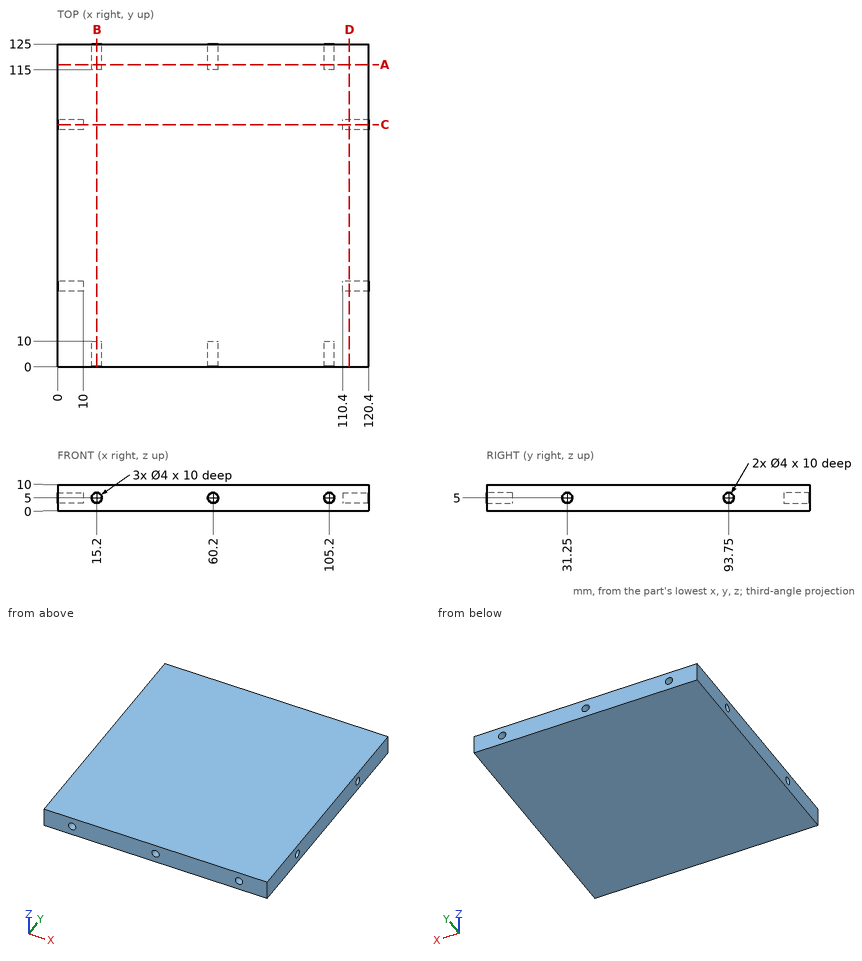
Could you check a few things on this drawing? It's one solid part, dimensions in mm from its lowest x, y, z. Give positions to 0.01 mm unless a question says otherwise; leave off trailing zeros. Write each loop counter-clockwise with the first axis right and the second up, starting at its lowest first coordinate (ties: lowest second). Pieces come first, ordered by that corner, then holes. Notation, with made-up numbers: (71, 0.25) -> (80, 0.25) arc R13 cw to (80, 22.25) -> close; hole circle Ø5 at (53.25, 78.5). An arc over 180 degrees is marked (long way). Answer as a JSON object with one key per item and string values.
Q1. Suppose I cut it at B-B on x = 15.2. Write out the boundary of the cut face in (y, z).
Taken from the geometry:
{"outline": "(0, 0) -> (125, 0) -> (125, 3) -> (115, 3) -> (115, 7) -> (125, 7) -> (125, 10) -> (0, 10) -> (0, 7) -> (10, 7) -> (10, 3) -> (0, 3) -> close"}
Q2. Will these pins go through, and if not, where does the flat tip stop? pin 1 Ø1.2 at (x, z) = (14.5, 4.5) entering from -Y; pin 2 Ø2 at (y, z) = (93, 4.5) entering from -X; pin 3 Ø1.2 at (x, z) = (106, 5.5) entering from +Y.
Taken from the geometry:
{"pin 1": "stops at y = 10", "pin 2": "stops at x = 10", "pin 3": "stops at y = 115"}
Q3. Suppose I cut it at D-D on x = 113. Write out the boundary of the cut face in (y, z), then the cut area to 3 significant figures.
Taken from the geometry:
{"outline": "(0, 0) -> (125, 0) -> (125, 10) -> (0, 10) -> close; hole circle Ø4 at (31.25, 5); hole circle Ø4 at (93.75, 5)", "area": "1,220 mm²"}
Q4. Please list where these lines run through material, in increasing order: L1, parallel to X at y = 3.5, z = 5; L2, parallel to Y at x = 7, z = 5; L3, parallel to Z at x = 105.2, y = 118.25.
Taken from the geometry:
{"L1": "x = 0 to 13.2, 17.2 to 58.2, 62.2 to 103.2, 107.2 to 120.4", "L2": "y = 0 to 29.25, 33.25 to 91.75, 95.75 to 125", "L3": "z = 0 to 3, 7 to 10"}
Q5. Suppose I cut it at A-A on y = 117. Write out the boundary of the cut face in (x, z).
Taken from the geometry:
{"outline": "(0, 0) -> (120.4, 0) -> (120.4, 10) -> (0, 10) -> close; hole circle Ø4 at (15.2, 5); hole circle Ø4 at (60.2, 5); hole circle Ø4 at (105.2, 5)"}
Q6. Suppose I cut it at C-C on y = 93.75. Write out the boundary of the cut face in (x, z), then the cut area to 3 significant figures.
Taken from the geometry:
{"outline": "(0, 0) -> (120.4, 0) -> (120.4, 3) -> (110.4, 3) -> (110.4, 7) -> (120.4, 7) -> (120.4, 10) -> (0, 10) -> (0, 7) -> (10, 7) -> (10, 3) -> (0, 3) -> close", "area": "1,120 mm²"}
